from build123d import *

# Parameters (mm, degrees)
SKETCH010_W         = 98.2
SKETCH010_H         = 60.1
PAD003002_DEPTH     = 1.6
SKETCH011_R         = 1.7
POCKET005002_DEPTH  = 1.601
SKETCH012_R         = 0.4
POCKET005003_DEPTH  = 1.601
LINEARPATTERN_COUNT = 16
LINEARPATTERN_PITCH = 2.54


with BuildPart() as part:
    # Sketch010 → Pad003002 (new body)
    with BuildSketch(Plane.XY):
        Rectangle(SKETCH010_W, SKETCH010_H)
    extrude(amount=-PAD003002_DEPTH)

    # Sketch011 (on Face5 of Pad003002) → Pocket005002 (cut, through all)
    with BuildSketch(Plane.XY):
        with Locations((-46.4, 27.35)):
            Circle(SKETCH011_R)
        with Locations((46.4, 27.35)):
            Circle(SKETCH011_R)
        with Locations((-46.4, -27.35)):
            Circle(SKETCH011_R)
        with Locations((46.4, -27.35)):
            Circle(SKETCH011_R)
    extrude(amount=-POCKET005002_DEPTH, mode=Mode.SUBTRACT)

    # Sketch012 (on Face4 of Pocket005002) → Pocket005003 (cut, through all)
    with BuildSketch(Plane.XY):
        with Locations((-38.9, 27.35)):
            Circle(SKETCH012_R)
    pocket005003 = extrude(amount=-POCKET005003_DEPTH, mode=Mode.SUBTRACT)

    # LinearPattern: Pocket005003 ×16
    with Locations(*[(i * LINEARPATTERN_PITCH, 0, 0) for i in range(1, LINEARPATTERN_COUNT)]):
        add(pocket005003, mode=Mode.SUBTRACT)


solid = part.part
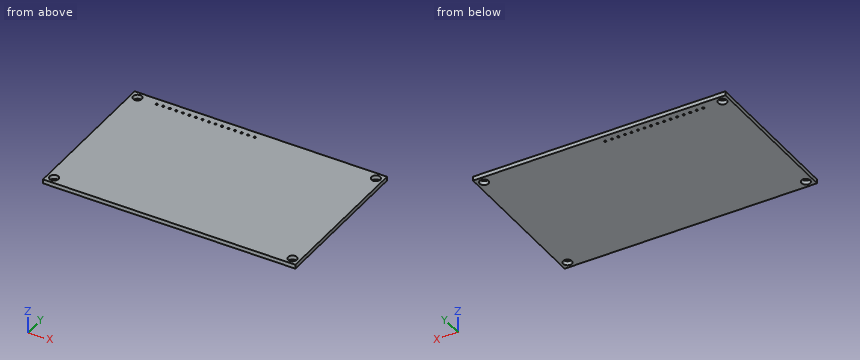
The model under review builds one solid part; all positions refer to its coordinate system, in mm. Give positions to 0.01 mm unless a question says otherwise; leave off trailing zeros. Order: outer loops, then holes, each group sorted by start corner. A loop starts at its lowest first (then second) coordinate and runs counter-clockwise, first axis right, second up. Notation, with made-up numbers: (-38.5, 73) -> (-2.5, 73) arc R33 ccw to (-2.5, 103) -> close; hole circle Ø10 at (15, 75.25). An arc over 180 degrees is marked (long way). Write item = value, one per line. Start each with the question number.
(1) Take a section at B-B (x = -46.4). Write out the cut boundary in (y, z).
(2) For L1, parallel to Y at x = -18.5, z = -0.9, list the stretches that pass through material, from the lowest coordinate up. Write a range as from..to.
(3) For pin 1 Ø2 at (x, y) = (-46.4, -27.35) entering from +Z, flat-tipped, find the tip position at first contact; note if it passes through.
(4) Take a section at A-A (y = -27.35). Write out the cut boundary in (x, z), plus the area to 3 significant figures.
Returned:
q1.outline = (-30.05, -1.6) -> (-29.05, -1.6) -> (-29.05, 0) -> (-30.05, 0) -> close; (-25.65, -1.6) -> (25.65, -1.6) -> (25.65, 0) -> (-25.65, 0) -> close; (29.05, -1.6) -> (30.05, -1.6) -> (30.05, 0) -> (29.05, 0) -> close
q2.L1 = -30.05..26.96, 27.74..30.05
q3.pin_1 = through
q4.outline = (-49.1, -1.6) -> (-48.1, -1.6) -> (-48.1, 0) -> (-49.1, 0) -> close; (-44.7, -1.6) -> (44.7, -1.6) -> (44.7, 0) -> (-44.7, 0) -> close; (48.1, -1.6) -> (49.1, -1.6) -> (49.1, 0) -> (48.1, 0) -> close
q4.area = 146 mm²
